CAD build for the part. Positions are in the model's coordinates, mm. Face numbers are marked on the shaded views. A direction names the side the tool comes from. Round coordinates to 2 decimals unless told otherwise and drop trailing zeros. Order: outer loops, then holes, each group sorted by start corner. A loop starts at its lowest first (then second) coordinate and runs counter-clockwise, first axis right, second up. Notation, with made-up numbers: (24, 56) - (50, 56) arc R12 cw to (50, 64) - close; hole circle Ø8 at (-13.5, 8). An arc over 180 degrees is marked (long way). Write item = value, one per line.
from build123d import *

# Parameters (mm, degrees)
SKETCH1_R           = 3
BOSS_EXTRUDE1_DEPTH = 10
SKETCH2_W           = 3
SKETCH2_H           = 2
CUT_EXTRUDE1_DEPTH  = 7
CHAMFER1_SIZE       = 0.5
FILLET1_R           = 0.5


with BuildPart() as part:
    # Sketch1 → Boss-Extrude1 (new body)
    with BuildSketch(Plane(origin=(0, 0, 0), x_dir=(1, 0, 0), z_dir=(0, 1, 0))):
        with Locations(Location((0, 0, 0), (0, 0, 270))):
            Circle(SKETCH1_R)
    extrude(amount=BOSS_EXTRUDE1_DEPTH)

    # Sketch2 → Cut-Extrude1 (cut)
    with BuildSketch(Plane.XZ):
        Rectangle(SKETCH2_W, SKETCH2_H)
    extrude(amount=-CUT_EXTRUDE1_DEPTH, mode=Mode.SUBTRACT)

    # Chamfer1
    chamfer1_edges = [part.edges().sort_by_distance(p)[0] for p in [
        (0, 0, -1),
        (0, 0, 1),
    ]]
    chamfer(chamfer1_edges, length=CHAMFER1_SIZE)

    # Fillet1
    fillet1_edges = [part.edges().sort_by_distance(p)[0] for p in [
        (0, 10, -3),
    ]]
    fillet(fillet1_edges, radius=FILLET1_R)


solid = part.part
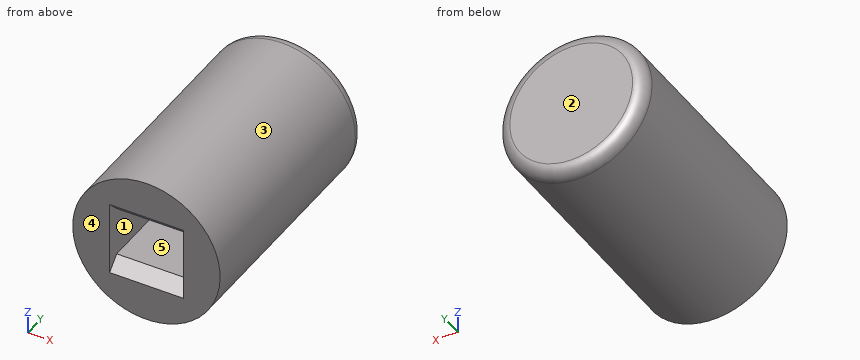
(1) Band-saw the part on A-A on z = 0. List the corners of the cut face in (x, y), plus the area to 3 significant figures.
Solved:
outline = (-3, 0) - (-1.5, 0) - (-1.5, 7) - (1.5, 7) - (1.5, 0) - (3, 0) - (3, 9.5) arc R0.5 ccw to (2.5, 10) - (-2.5, 10) arc R0.5 ccw to (-3, 9.5) - close
area = 38.9 mm²
(2) Drop a flat-ended pin along its axis: pin 1 (1 mm diameter, centred on x = 0.5, z = 0, fed in from -Y). Give the stop position or say it passes through.
Solved:
pin_1 = 7
(3) Band-saw the part on C-C on x = 0. List the corners of the cut face in (y, z), plus the area to 3 significant figures.
Solved:
outline = (0, -3) - (9.5, -3) arc R0.5 ccw to (10, -2.5) - (10, 2.5) arc R0.5 ccw to (9.5, 3) - (0, 3) - (0, 1.5) - (0.5, 1) - (7, 1) - (7, -1) - (0.5, -1) - (0, -1.5) - close
area = 45.6 mm²
(4) Band-saw the part on B-B on y = 1.25. List the corners of the cut face in (x, z), plus the area to 3 significant figures.
Solved:
outline = circle Ø6 at (0, 0); hole (-1.5, -1) - (1.5, -1) - (1.5, 1) - (-1.5, 1) - close
area = 22.3 mm²
(5) Probe line 1 along Z through (x, y) = (-0.05, 1.75); line 2 along X through (y, z) = (2, -0.7); line 3 along Y through (x, z) = (0.75, -0.7). List the from-to ranges inside material, lowest first.
Solved:
line_1 = -3 to -1, 1 to 3
line_2 = -2.92 to -1.5, 1.5 to 2.92
line_3 = 7 to 10
(6) Band-saw the part on D-D on y = 8.5. List the corners of the cut face in (x, z), plus the area to 3 significant figures.
Solved:
outline = circle Ø6 at (0, 0)
area = 28.3 mm²
(7) Tool access for the marked faces 4 and 5: list every direction of +Z, -Z, +X, -X, +Y, -Y with a clear straight run to the whole face (end or side of a thin tool).
Solved:
face_4 = +Z, -Z, +X, -X, -Y
face_5 = -Y
(8) Pull direction X, two halves, no side cores. Call the marked faces 1, 2 and 3: released by +X, released by -X, zero draft, split by the parting line, or undercut.
Solved:
face_1 = undercut
face_2 = zero draft
face_3 = split by the parting line
